from build123d import *

# Parameters (mm, degrees)
SKETCH1_W               = 76.2
SKETCH1_H               = 25.4
SKETCH1_W_2             = 69.85
SKETCH1_H_2             = 19.05
BOSS_EXTRUDE1_DEPTH     = 177.8
SKETCH2_R               = 25
CUT_EXTRUDE1_DEPTH      = 184.601770144
CUT_EXTRUDE2_DEPTH      = 194.857086535
CUT_EXTRUDE2_DEPTH_BACK = 194.857086535
SKETCH3_R               = 4.7625
CUT_EXTRUDE3_DEPTH      = 184.601770144
CUT_EXTRUDE3_DEPTH_BACK = 184.601770144
SKETCH4_R               = 3.175


with BuildPart() as part:
    # Sketch1 → Boss-Extrude1 (new body)
    with BuildSketch(Plane(origin=(0, 0, 0), x_dir=(1, 0, 0), z_dir=(0, 1, 0))):
        Rectangle(SKETCH1_W, SKETCH1_H)
        Rectangle(SKETCH1_W_2, SKETCH1_H_2, mode=Mode.SUBTRACT)
    extrude(amount=BOSS_EXTRUDE1_DEPTH)

    # Sketch2 → Cut-Extrude1 (cut, through all)
    with BuildSketch(Plane.XY.offset(12.7)):
        with Locations((0, 146.05)):
            Circle(SKETCH2_R)
    extrude(amount=-CUT_EXTRUDE1_DEPTH, mode=Mode.SUBTRACT)

    # Sketch3 → Cut-Extrude2 (cut, two sides: drawn at the far end of the back side and taken through both)
    with BuildSketch(Plane.ZY.offset(38.1).offset(-CUT_EXTRUDE2_DEPTH_BACK)):
        with Locations((0, 146.05)):
            Circle(SKETCH3_R)
    extrude(amount=CUT_EXTRUDE2_DEPTH + CUT_EXTRUDE2_DEPTH_BACK, mode=Mode.SUBTRACT)

    # Sketch4 → Cut-Extrude3 (cut, two sides: drawn at the far end of the back side and taken through both)
    with BuildSketch(Plane.XY.offset(12.7).offset(-CUT_EXTRUDE3_DEPTH_BACK)):
        with Locations((-19.05, 66.675)):
            Circle(SKETCH4_R)
        with Locations((19.05, 66.675)):
            Circle(SKETCH4_R)
        with Locations((19.05, 22.225)):
            Circle(SKETCH4_R)
        with Locations((-19.05, 22.225)):
            Circle(SKETCH4_R)
    extrude(amount=CUT_EXTRUDE3_DEPTH + CUT_EXTRUDE3_DEPTH_BACK, mode=Mode.SUBTRACT)


solid = part.part
Geometry: final body of the model. Coordinates: model frame, mm. A direction names the side the tool comes from. Coordinates: 2 decimals unless noted, no trailing zeros. Loops run counter-clockwise (first coordinate to the right, second up) from the corner with the lowest first, then second, coordinate; pieces in that order, holes last. Notation, with made-up numbers: (40.25, 66.25) - (53.25, 66.25) arc R27 ccw to (53.25, 98.25) - close; hole circle Ø2 at (21.5, 56.25). An arc over 180 degrees is marked (long way). One line per question, with ' | ' between items. Start each with the question number.
(1) Reachability of faces 4 (the cylindrical face through (16.53, 64.743, 11.09)), 5 (the flat face through (34.925, 88, 0)) from +Z, -Z, +X, -X, +Y, -Y: full face, straight path, thin tool, end or side. Return the list, or none.
(2) Ray query, L1, parallel to X at y = 38, z = 4 (3 decimals); L2, parallel to Z at x = 32, y = 12 (3 decimals); L3, parallel to Y at x = 19.05, z = -10.35. Return the intervals inside material, ascending. Write a range as from..to.
(3) Cut plane A-A on y = 146.05. Output: boundary loops of the cut face in (x, z) (1 decimal), and give its area (3 significant figures).
(4) Draft query along Y for faces 1 (the cylindrical face through (-3.255, 170.837, -11.09)), 2 (the flat face through (-3, 177.8, 10)), 3 (the flat face through (-1, 68, -12.7)). Return one class per face: +Y half, -Y half, draft (parallel to the pull), parting line (faces both ways), or undercut.
(5) Cut plane B-B on x = 12.5. Output: boundary loops of the cut face in (y, z) (3 decimals).
(6) First-contact query: pin 1 (10 mm diameter, centred on x = -19.05, y = 66.675, fed in from -Z). Flat tip, straight axial feed; report the tip coordinate or a pass-through.
(7) Cut plane C-C on z = 0. Output: boundary loops of the cut face in (x, y) (1 decimal).
(8) Cut plane D-D on y = 36.5. Output: boundary loops of the cut face in (x, z) (3 decimals).
Here are the results:
1) face 4: +Z, -Z | face 5: +Y, -Y
2) L1: -38.1..-34.925, 34.925..38.1 | L2: -12.7..-9.525, 9.525..12.7 | L3: 0..19.05, 25.4..63.5, 69.85..129.86, 162.24..177.8
3) outline: (-38.1, -12.7) - (-25, -12.7) - (-25, -9.5) - (-34.9, -9.5) - (-34.9, -4.8) - (-38.1, -4.8) - close; (-38.1, 4.8) - (-34.9, 4.8) - (-34.9, 9.5) - (-25, 9.5) - (-25, 12.7) - (-38.1, 12.7) - close; (25, -12.7) - (38.1, -12.7) - (38.1, -4.8) - (34.9, -4.8) - (34.9, -9.5) - (25, -9.5) - close; (25, 9.5) - (34.9, 9.5) - (34.9, 4.8) - (38.1, 4.8) - (38.1, 12.7) - (25, 12.7) - close | area: 227 mm²
4) face 1: undercut | face 2: +Y half | face 3: draft
5) outline: (0, -12.7) - (124.399, -12.7) - (124.399, -9.525) - (0, -9.525) - close; (0, 9.525) - (124.399, 9.525) - (124.399, 12.7) - (0, 12.7) - close; (167.701, -12.7) - (177.8, -12.7) - (177.8, -9.525) - (167.701, -9.525) - close; (167.701, 9.525) - (177.8, 9.525) - (177.8, 12.7) - (167.701, 12.7) - close
6) pin 1: z = -12.7
7) outline: (-38.1, 0) - (-34.9, 0) - (-34.9, 141.3) - (-38.1, 141.3) - close; (-38.1, 150.8) - (-34.9, 150.8) - (-34.9, 177.8) - (-38.1, 177.8) - close; (34.9, 0) - (38.1, 0) - (38.1, 141.3) - (34.9, 141.3) - close; (34.9, 150.8) - (38.1, 150.8) - (38.1, 177.8) - (34.9, 177.8) - close
8) outline: (-38.1, -12.7) - (38.1, -12.7) - (38.1, 12.7) - (-38.1, 12.7) - close; hole (-34.925, -9.525) - (34.925, -9.525) - (34.925, 9.525) - (-34.925, 9.525) - close
